```python
from build123d import *

# Parameters (mm, degrees)
SKETCH_1_R                     = 1.45
SHANK_THREADS_SIMPLIFIED_DEPTH = 12
SKETCH_2_R                     = 2.75
HEAD_DEPTH                     = 3
HEX_SOCKET_DEPTH               = 1.95


with BuildPart() as part:
    # 草图1 → Shank_threads_simplified (new body)
    with BuildSketch(Plane.XY):
        Circle(SKETCH_1_R)
    extrude(amount=-SHANK_THREADS_SIMPLIFIED_DEPTH)

    # 草图2 → Head (add)
    with BuildSketch(Plane.XY):
        Circle(SKETCH_2_R)
    extrude(amount=HEAD_DEPTH)

    # 草图3 → Hex_socket (cut)
    with BuildSketch(Plane.XY.offset(3)):
        Polygon((1.25, 0.721687836), (0, 1.443375673), (-1.25, 0.721687836), (-1.25, -0.721687836), (0, -1.443375673), (1.25, -0.721687836), align=None)
    extrude(amount=-HEX_SOCKET_DEPTH, mode=Mode.SUBTRACT)


solid = part.part
```
Input: part model. Units: mm. Frame: model coordinates. A direction names the side the tool comes from. Coordinates: 2 decimals unless noted, no trailing zeros. Write each loop counter-clockwise with the first axis right and the second up, starting at its lowest first coordinate (ties: lowest second). Pieces come first, ordered by that corner, then holes.
1) Material intervals for line 1 along Z through (x, y) = (1.45, -1.3); line 2 along Y through (x, z) = (0.05, -2); line 3 along Z through (x, y) = (0.25, -0.25), sorted ascending.
2) Section C-C on z = -5. Output: boundary loops of the cut face in (x, y), and give its area (3 significant figures).
3) Section A-A on y = 0. Output: boundary loops of the cut face in (x, z), and give its area (3 significant figures).
4) Pin query (flat end, axial travel): pin 1 Ø2 at (y, z) = (-1.5, -0.5) entering from +X; pin 2 Ø1.5 at (x, z) = (-1.5, -4.5) entering from -Y. Return the tip coordinate at first contact, or that it passes through.
5) Mould query, pull axis X, two halves, no side actions, for faces 4 (the flat face through (0, 0, -12)), 5 (the cylindrical face through (-1.45, 0.06, -5.92)), 6 (the flat face through (-0.616, 1.088, 2.039)). Classes: pulls with the +X half, pulls with the -X half, needs draft (parallel to the pull), parting line crosses it, or undercut.
6) Set-up query: faces 1 (the flat face through (-1.25, 0, 2)), 2 (the cylindrical face through (-0.596, -2.685, 1.479)), 3 (the flat face through (1.2, -1.2, 0)). Return all of +Z, -Z, +X, -X, +Y, -Y with unobstructed straight access to the full face (end or side cutting, diameter ignored); none if empty.
7) Section B-B on x = -1.05. Output: boundary loops of the cut face in (y, z).
8) Section D-D on y = -2. Output: boundary loops of the cut face in (x, z).
Check result:
1. line 1: z = 0 to 3
1. line 2: y = -1.45 to 1.45
1. line 3: z = -12 to 1.05
2. outline: circle Ø2.9 at (0, 0)
2. area: 6.61 mm2
3. outline: (-2.75, 0) - (-1.45, 0) - (-1.45, -12) - (1.45, -12) - (1.45, 0) - (2.75, 0) - (2.75, 3) - (1.25, 3) - (1.25, 1.05) - (-1.25, 1.05) - (-1.25, 3) - (-2.75, 3) - close
3. area: 46.4 mm2
4. pin 1: stops at x = 2.68
4. pin 2: stops at y = -1.24
5. face 4: needs draft
5. face 5: parting line crosses it
5. face 6: undercut
6. face 1: +Z
6. face 2: +Z, -Z
6. face 3: -Z
7. outline: (-2.54, 0) - (-1, 0) - (-1, -12) - (1, -12) - (1, 0) - (2.54, 0) - (2.54, 3) - (0.84, 3) - (0.84, 1.05) - (-0.84, 1.05) - (-0.84, 3) - (-2.54, 3) - close
8. outline: (-1.89, 0) - (1.89, 0) - (1.89, 3) - (-1.89, 3) - close
